from build123d import *

# Parameters (mm, degrees)
BOSS_EXTRUDE1_START = -352.453482
SKETCH1_R           = 23.525
SKETCH1_R_2         = 22.525
BOSS_EXTRUDE1_DEPTH = 20
BOSS_EXTRUDE2_DEPTH = 40
SKETCH3_R           = 18
CUT_EXTRUDE1_DEPTH  = 74.525


with BuildPart() as part:
    # Sketch1 → Boss-Extrude1 (new body, symmetric)
    with BuildSketch(Plane.XY.offset(BOSS_EXTRUDE1_START)):
        Circle(SKETCH1_R)
        Circle(SKETCH1_R_2, mode=Mode.SUBTRACT)
    extrude(amount=BOSS_EXTRUDE1_DEPTH, both=True)

    # Sketch4 → Boss-Extrude2 (add)
    with BuildSketch(Plane.XY.offset(-332.453482287)):
        Polygon((23.525, -23.525), (23.525, -24.525), (-23.525, -24.525), (-23.525, -23.525), (0, -23.525), align=None)
        with BuildLine():
            ThreePointArc((0, -23.525), (-16.634687027, -16.634687027), (-23.525, 0))
            Line((-23.525, 0), (-23.525, -23.525))
            Line((-23.525, -23.525), (0, -23.525))
        make_face()
        with BuildLine():
            Line((23.525, -23.525), (23.525, 0))
            ThreePointArc((23.525, 0), (16.634687027, -16.634687027), (0, -23.525))
            Line((0, -23.525), (23.525, -23.525))
        make_face()
    extrude(amount=-BOSS_EXTRUDE2_DEPTH)

    # Sketch3 → Cut-Extrude1 (cut, through all)
    with BuildSketch(Plane.XZ.offset(50)):
        with Locations((0, -352.453482287)):
            Circle(SKETCH3_R)
    extrude(amount=-CUT_EXTRUDE1_DEPTH, mode=Mode.SUBTRACT)


solid = part.part
Input: part model. Units: mm. Frame: model coordinates. Give positions to 0.01 mm unless a question says otherwise; leave off trailing zeros. Write each loop counter-clockwise with the first axis right and the second up, starting at its lowest first coordinate (ties: lowest second). Pieces come first, ordered by that corner, then holes.
Q1. Section D-D, the plane x = -5.5. Output: boundary loops of the cut face in (y, z) (3 decimals).
Q2. Pull-direction query (Y, two-part tool) for faces 1 (the face through (-23.525, -12, -352)), 2 (the face through (20.63, 11.31, -352.17)), 3 (the face through (-17.875, -13.706, -357.178)); classes: pulls with the +Y half, pulls with the -Y half, needs draft (parallel to the pull), parting line crosses it, or undercut.
Q3. Section A-A, the plane x = 0. Output: boundary loops of the cut face in (y, z) (3 decimals), plus the area to 3 significant figures.
Q4. Section B-B, the plane y = 7.5. Output: boundary loops of the cut face in (x, z), plus the area to 3 significant figures.
Q5. Material intervals for probe 1 along X at (y, z) = (0.5, -344); probe 2 along X at (y, z) = (-3, -359) (3 decimals); probe 3 along Y at (x, z) = (-19, -356.5) (3 decimals), sorted ascending.
Q6. First-contact query: P1, Ø4, axis at y = 14.5, z = -355, coming from the +X side. Flat tip, straight axial feed; report the tip coordinate or a pass-through.
Q7. Section C-C, the plane z = -365.5. Output: boundary loops of the cut face in (x, y) (3 decimals).
Filled in:
1. outline: (-24.525, -372.453) - (-21.843, -372.453) - (-21.843, -369.593) - (-24.525, -369.593) - close; (-24.525, -335.314) - (-21.843, -335.314) - (-21.843, -332.453) - (-24.525, -332.453) - close; (21.843, -372.453) - (22.873, -372.453) - (22.873, -369.593) - (21.843, -369.593) - close; (21.843, -335.314) - (22.873, -335.314) - (22.873, -332.453) - (21.843, -332.453) - close
2. face 1: needs draft
2. face 2: pulls with the +Y half
2. face 3: undercut
3. outline: (-24.525, -372.453) - (-22.525, -372.453) - (-22.525, -370.453) - (-24.525, -370.453) - close; (-24.525, -334.453) - (-22.525, -334.453) - (-22.525, -332.453) - (-24.525, -332.453) - close; (22.525, -372.453) - (23.525, -372.453) - (23.525, -370.453) - (22.525, -370.453) - close; (22.525, -334.453) - (23.525, -334.453) - (23.525, -332.453) - (22.525, -332.453) - close
3. area: 12.0 mm2
4. outline: (-22.3, -372.45) - (-21.24, -372.45) - (-21.24, -332.45) - (-22.3, -332.45) - close; (21.24, -372.45) - (22.3, -372.45) - (22.3, -332.45) - (21.24, -332.45) - close
4. area: 84.6 mm2
5. probe 1: x = -23.52 to -22.52, 22.52 to 23.52
5. probe 2: x = -23.525 to -22.324, 22.324 to 23.525
5. probe 3: y = -24.525 to -12.099, 12.099 to 13.872
6. P1: stops at x = 19.93
7. outline: (-23.525, -24.525) - (-12.401, -24.525) - (-12.401, -18.804) arc R22.525 cw to (-12.401, 18.804) - (-12.401, 19.991) arc R23.525 ccw to (-23.525, 0) - close; (12.401, -24.525) - (23.525, -24.525) - (23.525, 0) arc R23.525 ccw to (12.401, 19.991) - (12.401, 18.804) arc R22.525 cw to (12.401, -18.804) - close
